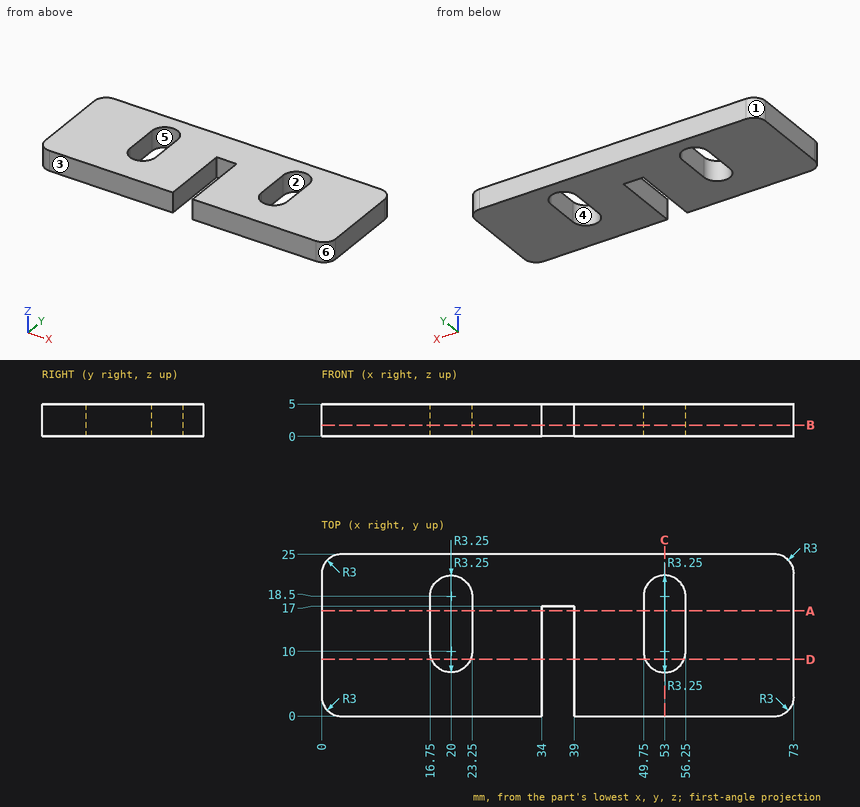
Source: three-view drawing plus pictorial views. Frame: mm from the lowest corner of the part. A direction names the side the tool comes from. Round coordinates to 2 decimals unless told otherwise and drop trailing zeros. Loops run counter-clockwise (first coordinate to the right, second up) from the corner with the lowest first, then second, coordinate; pieces in that order, holes last.
Q1. Mould query, pull axis X, two halves, no side actions, for the marked faces 3, 4, 5 and 6. Classes: pulls with the +X half, pulls with the -X half, needs draft (parallel to the pull), parting line crosses it, or undercut.
Q2. Access query for the marked faces 1 and 2. Directions: +Z, -Z, +X, -X, +Y, -Y. A direction counts if a zero-diameter tool reaches every point of the face in a straight line with its end or side. Return the directions, or none.
Q3. Section A-A, the plane y = 16.25. Return loops of the section in (x, z), plus the area to 3 significant figures.
Q4. Section B-B, the plane z = 1.75. Return loops of the section in (x, y), plus the area to 3 significant figures.
Q5. Section C-C, the plane x = 53. Return loops of the section in (y, z), plus the area to 3 significant figures.
Q6. First-contact query: P1, Ø2, axis at x = 24, y = 8, coming from the -Z side; P2, Ø2.5, axis at x = 37.5, z = 2, coming from the -Y side. Flat tips, straight axial feed; report the tip coordinate or a pass-through.
Q7. Ray query, line 1 (X direction, y = 11.5, z = 0.6); line 2 (X direction, y = 17.5, z = 4.25); line 3 (X direction, y = 7.25, z = 4.3). Return the intervals inside material, ascending.
Q8. Section D-D, the plane y = 8.75. Return loops of the section in (x, z).
Solutions:
1. face 3: needs draft
1. face 4: undercut
1. face 5: undercut
1. face 6: pulls with the +X half
2. face 1: +Z, -Z, -X, +Y
2. face 2: +Z, -Z
3. outline: (0, 0) - (16.75, 0) - (16.75, 5) - (0, 5) - close; (23.25, 0) - (34, 0) - (34, 5) - (23.25, 5) - close; (39, 0) - (49.75, 0) - (49.75, 5) - (39, 5) - close; (56.25, 0) - (73, 0) - (73, 5) - (56.25, 5) - close
3. area: 275 mm2
4. outline: (0, 3) arc R3 ccw to (3, 0) - (34, 0) - (34, 17) - (39, 17) - (39, 0) - (70, 0) arc R3 ccw to (73, 3) - (73, 22) arc R3 ccw to (70, 25) - (3, 25) arc R3 ccw to (0, 22) - close; hole (16.75, 10) arc R3.25 ccw to (23.25, 10) - (23.25, 18.5) arc R3.25 ccw to (16.75, 18.5) - close; hole (49.75, 10) arc R3.25 ccw to (56.25, 10) - (56.25, 18.5) arc R3.25 ccw to (49.75, 18.5) - close
4. area: 1,560 mm2
5. outline: (0, 0) - (6.75, 0) - (6.75, 5) - (0, 5) - close; (21.75, 0) - (25, 0) - (25, 5) - (21.75, 5) - close
5. area: 50.0 mm2
6. P1: stops at z = 0
6. P2: stops at y = 17
7. line 1: x = 0 to 16.75, 23.25 to 34, 39 to 49.75, 56.25 to 73
7. line 2: x = 0 to 16.75, 23.25 to 49.75, 56.25 to 73
7. line 3: x = 0 to 18.27, 21.73 to 34, 39 to 51.27, 54.73 to 73
8. outline: (0, 0) - (17, 0) - (17, 5) - (0, 5) - close; (23, 0) - (34, 0) - (34, 5) - (23, 5) - close; (39, 0) - (50, 0) - (50, 5) - (39, 5) - close; (56, 0) - (73, 0) - (73, 5) - (56, 5) - close
